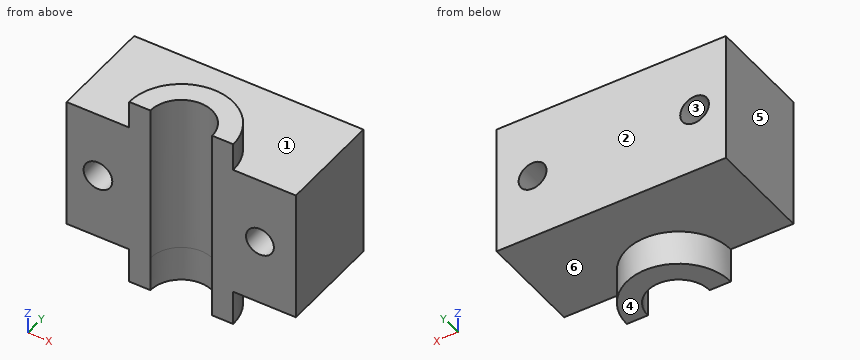
from build123d import *

# Parameters (mm, degrees)
F0_W          = 128.197401762
F0_H          = 73.774009943
F1_DEPTH      = 58.42
F2_DEPTH      = 19.5215027779
F2_DEPTH_BACK = 89.3221944571
F7_R          = 17.2672830395
F3_DEPTH      = 89.3231944571
F3_DEPTH_BACK = 25.4
F8_R          = 7.783506766
F4_DEPTH      = 58.421
F9_R          = 8.0252632598
F10_DEPTH     = 58.421


with BuildPart() as f1:
    # F0 (on Front) → F1 (new body)
    with BuildSketch(Plane.XZ):
        Rectangle(F0_W, F0_H)
    extrude(amount=F1_DEPTH)

    # F6 (on face) → F2 (join, two sides)
    with BuildSketch(Plane(origin=(0, 0, -36.8870049715), x_dir=(1, 0, 0), z_dir=(0, 0, -1))) as f2_sk:
        with BuildLine():
            ThreePointArc((-29.0746443466, 58.42), (0, 29.3453556534), (29.0746443466, 58.42))
            Line((29.0746443466, 58.42), (-29.0746443466, 58.42))
        make_face()
    extrude(amount=F2_DEPTH)
    extrude(f2_sk.sketch, amount=-F2_DEPTH_BACK)

    # F7 (on face) → F3 (cut, two sides)
    with BuildSketch(Plane(origin=(0, 0, -36.8870049715), x_dir=(1, 0, 0), z_dir=(0, 0, -1))) as f3_sk:
        with Locations((0, 58.42)):
            Circle(F7_R)
    extrude(amount=-F3_DEPTH, mode=Mode.SUBTRACT)
    extrude(f3_sk.sketch, amount=F3_DEPTH_BACK, mode=Mode.SUBTRACT)

    # F8 (on face) → F4 (cut, through all)
    with BuildSketch(Plane.XZ.offset(58.42)):
        with Locations((44.0028309822, 0)):
            Circle(F8_R)
    extrude(amount=-F4_DEPTH, mode=Mode.SUBTRACT)

    # F9 (on face) → F10 (cut, through all)
    with BuildSketch(Plane.XZ.offset(58.42)):
        with Locations((-46.5866726138, 0)):
            Circle(F9_R)
    extrude(amount=-F10_DEPTH, mode=Mode.SUBTRACT)


solid = f1.part
Geometry check sheet. Reference: the model listing, model coordinates, mm. Face numbers are marked on the shaded views. A direction names the side the tool comes from. Round coordinates to 2 decimals unless told otherwise and drop trailing zeros. Order: outer loops, then holes, each group sorted by start corner. A loop starts at its lowest first (then second) coordinate and runs counter-clockwise, first axis right, second up. Notation, with made-up numbers: M 46.5,71 L 70.5,71 A20 cw 70.5,92 Z; hole C 71.25,-23 d7. An arc over 180 degrees is marked long. Answer in a Markdown table with one row per item. Add a question column.
Item 1: Sectioned sample at B-B, the plane y = -21. Enter the section's corners in (x, z).
Item 2: Material ranges on L1, parallel to X at y = -5.5, z = 0.5; L2, parallel to Z at x = -48.5, y = -26.5; L3, parallel to Z at x = -14, y = -22.5, recorded low to high. Write a range as [from, to].
Item 3: Set-up check for the marked faces 5 and 6: record each of +Z, -Z, +X, -X, +Y, -Y from which the full face is reachable in a straight line by a thin tool's end or side.
Item 4: Sectioned sample at A-A, the plane z = 0. Enter the section's corners in (x, y).
Item 5: Sectioned sample at C-C, the plane x = -43.5. Enter the section's corners in (y, z).
Item 6: Draft check along Z on the marked faces 1, 2, 3 and 4. Enter one of: released by +Z, released by -Z, zero draft, split by the parting line, or undercut.
Item 7: Sectioned sample at D-D, the plane z = 31. Enter the section's corners in (x, y).
Item 8: Depth check by flat-ended pin: pin 1 Ø6 at (x, z) = (9, -3.5) entering from -Y; pin 2 Ø10 at (x, z) = (4.5, 25) entering from +Y; pin 3 Ø4 at (x, z) = (14, 2) entering from -Y; pin 4 Ø2 at (x, y) = (-22, -25) entering from -Z. Enter the tip coordinate at first touch or a pass-through.
Filled in:
| question | item | result |
|---|---|---|
| 1 | outline | M -64.1,-36.89 L 64.1,-36.89 L 64.1,36.89 L -64.1,36.89 Z; hole C -46.59,0 d16.05; hole C 44,0 d15.57 |
| 2 | L1 | x = [-64.1, -54.6], [-38.58, 36.24], [51.77, 64.1] |
| 2 | L2 | z = [-36.89, -7.79], [7.79, 36.89] |
| 2 | L3 | z = [-36.89, 36.89] |
| 3 | face 5 | +Z, -Z, -X, +Y, -Y |
| 3 | face 6 | -Z, +Y |
| 4 | outline | M -64.1,-58.42 L -54.61,-58.42 L -54.61,0 L -64.1,0 Z; M -38.56,-58.42 L -17.27,-58.42 A17.27 cw 17.27,-58.42 L 36.22,-58.42 L 36.22,0 L -38.56,0 Z; M 51.79,-58.42 L 64.1,-58.42 L 64.1,0 L 51.79,0 Z |
| 5 | outline | M -58.42,-36.89 L 0,-36.89 L 0,-7.41 L -58.42,-7.41 Z; M -58.42,7.41 L 0,7.41 L 0,36.89 L -58.42,36.89 Z |
| 6 | face 1 | released by +Z |
| 6 | face 2 | zero draft |
| 6 | face 3 | undercut |
| 6 | face 4 | released by -Z |
| 7 | outline | M -64.1,-58.42 L -17.27,-58.42 A17.27 cw 17.27,-58.42 L 64.1,-58.42 L 64.1,0 L -64.1,0 Z |
| 8 | pin 1 | stops at y = -46 |
| 8 | pin 2 | stops at y = 0 |
| 8 | pin 3 | stops at y = -51.93 |
| 8 | pin 4 | stops at z = -36.89 |
